Autodesk Inventor part; units mm, degrees
ref_plane "YZ Plane" through (0, 0, 0) normal (1, 0, 0) x (0, 1, 0)
ref_plane "XZ Plane" through (0, 0, 0) normal (0, 1, 0) x (-1, 0, 0)
ref_plane "XY Plane" through (0, 0, 0) normal (0, 0, 1) x (1, 0, 0)
sketch "Sketch3" plane through (0, 0, 0) normal (0, 0, 1) x (1, 0, 0)
  line L0 (-12.7, -19.05) -> (12.7, -19.05)
  line L1 (12.7, -19.05) -> (12.7, 19.05)
  line L2 (12.7, 19.05) -> (-12.7, 19.05)
  line L3 (-12.7, 19.05) -> (-12.7, -19.05)
  line L4 (-12.7, -19.05) -> (12.7, 19.05) construction
  line L5 (12.7, -19.05) -> (-12.7, 19.05) construction
  point P0 (0, 0)
  dimension "d0" = 25.4
  dimension "d1" = 38.1
extrude "Extrusion1" add sketch "Sketch3" along normal mid plane 12.7
sketch "Sketch4" plane through (0, 0, 6.35) normal (0, 0, 1) x (1, 0, 0)
  circle A0 centre (0, 0) radius 2.667
  dimension "d4" = 5.334
extrude "Extrusion2" cut sketch "Sketch4" against normal through all
sketch "Sketch5" plane through (-12.7, -19.05, 6.35) normal (-1, 0, 0) x (0, 0, 1)
  line L0 (3.175, 6.35) -> (50.8, 6.35)
  line L1 (-12.7, 38.1) -> (-12.7, 0)
  line L2 (0, 0) -> (0, 38.1)
  line L3 (-12.7, 0) -> (0, 0)
  line L4 (0, 0) -> (0, 6.35)
  line L5 (0, 6.35) -> (-12.7, 6.35)
  line L6 (-12.7, 6.35) -> (-12.7, 0)
  point P0 (-6.35, 19.05)
  point P1 (-12.7, 6.35)
  dimension "d9" = 6.35
extrude "Extrusion3" cut sketch "Sketch5" against normal through all
sketch "Sketch8" plane through (-12.7, -12.7, -6.35) normal (-1, 0, 0) x (0, 0, 1)
  line L0 (-4.7625, 21.8398) -> (-4.7625, 13.2284)
  line L1 (12.7, 0) -> (12.7, 31.75)
  line L2 (12.7, 0) -> (-4.7625, 0)
  line L3 (-4.7625, 0) -> (-4.7625, 31.75)
  line L4 (-4.7625, 31.75) -> (12.7, 31.75)
  line L5 (12.7, 31.75) -> (12.7, 0)
  point P0 (6.35, 12.7)
  point P1 (-4.7625, 13.2284)
extrude "Extrusion5" add sketch "Sketch8" along normal blind 6.35
mirror "Mirror1" about plane through (0, 0, 0) normal (1, 0, 0) of "Extrusion5"
sketch "Sketch6" plane through (0, 0, 0) normal (0, 0, 1) x (1, 0, 0)
  circle A0 centre (0, 25.4) radius 15.367
  point P0 (0, 0)
  dimension "d10" = 25.4
  dimension "d13" = 30.734
extrude "cutOutForGuide" cut sketch "Sketch6" along normal mid plane 11.0998
sketch "Sketch9" plane through (0, 0, 6.35) normal (0, 0, 1) x (1, 0, 0)
  circle A0 centre (0, 0) radius 3.1242
  dimension "d16" = 6.2484
extrude "Extrusion6" cut sketch "Sketch9" against normal blind 9.525
properties part number "preventWireJumpingSingleSupport" material "PBT Plastic"
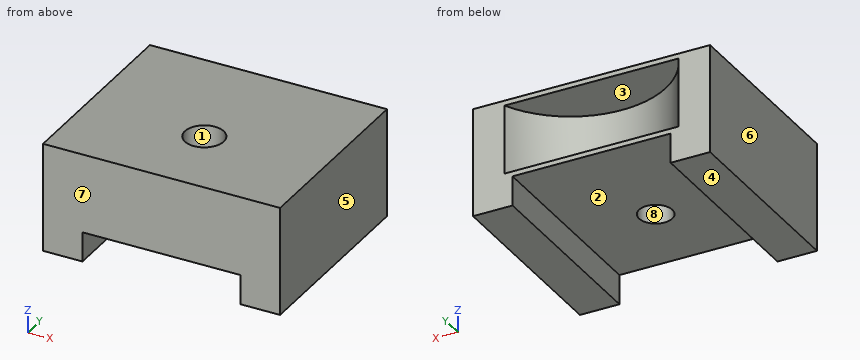
CAD build for the part. Positions are in the model's coordinates, mm. Face numbers are marked on the shaded views. A direction names the side the tool comes from. Round coordinates to 2 decimals unless told otherwise and drop trailing zeros. Write each loop counter-clockwise with the first axis right and the second up, starting at its lowest first coordinate (ties: lowest second). Pieces come first, ordered by that corner, then holes. Notation, with made-up numbers: (21.5, 8.25) - (40.5, 8.25) arc R15 cw to (40.5, 25.25) - close; hole circle Ø9 at (-27, 67). An arc over 180 degrees is marked (long way). Return JSON: item names as keys, results as strings. Group by question number.
Item 1: Mould opens along X. For the marked faces 5, 6, 7 and 8 say: +X half, -X half, draft (parallel to the pull), parting line (faces both ways), or undercut.
Item 2: Band-saw the part on D-D on z = -7.5. List the corners of the cut face in (x, y).
Item 3: Band-saw the part on C-C on z = -3.75. List the corners of the cut face in (x, y).
Item 4: Band-saw the part on A-A on x = 0. List the corners of the cut face in (y, z) (3 decimals).
Item 5: 3-axis set-ups, long thin cutter, end or side, ignore diameter. For the marked faces 1, 2, 3 and 4: which of +Z, -Z, +X, -X, +Y, -Y reach the whole face in a straight line?
Item 6: Probe probe 1 along Y at (x, z) = (0, 4.25); probe 2 along Z at (x, y) = (-3.5, -4); probe 3 along Y at (x, z) = (0, -4.75). List the from-to ranges inside material, lowest first.
Item 7: Flat gauge pins, fed straight in: pin 1 Ø3 at (x, z) = (-4.5, 0.5) entering from +Y; pin 2 Ø7 at (x, y) = (2, 16.5) entering from -Z; pin 3 Ø10 at (x, z) = (3, -0.5) entering from +Y. Where does each tip first touch, or does it go through?
Resolved:
{
 "1": {"face 5": "+X half", "face 6": "-X half", "face 7": "draft", "face 8": "undercut"},
 "2": {"outline": "(-19.05, -12.7) - (-12.7, -12.7) - (-12.7, 19.05) - (-19.05, 19.05) - close; (12.7, -12.7) - (19.05, -12.7) - (19.05, 19.05) - (12.7, 19.05) - close"},
 "3": {"outline": "(-19.05, -12.7) - (19.05, -12.7) - (19.05, 19.05) - (13.99, 19.05) arc R15.37 cw to (-13.99, 19.05) - (-19.05, 19.05) - close; hole circle Ø5.33 at (0, 0)"},
 "4": {"outline": "(-12.7, -6.35) - (-2.667, -6.35) - (-2.667, -3.175) - (-3.124, -3.175) - (-3.124, 6.35) - (-12.7, 6.35) - close; (2.667, -6.35) - (19.05, -6.35) - (19.05, -5.55) - (10.033, -5.55) - (10.033, 5.55) - (19.05, 5.55) - (19.05, 6.35) - (3.124, 6.35) - (3.124, -3.175) - (2.667, -3.175) - close"},
 "5": {"face 1": "+Z", "face 2": "-Z, +Y, -Y", "face 3": "+Y", "face 4": "-Z, +X, -X, +Y, -Y"},
 "6": {"probe 1": "y = -12.7 to -3.12, 3.12 to 10.03", "probe 2": "z = -6.35 to 6.35", "probe 3": "y = -12.7 to -2.67, 2.67 to 10.03"},
 "7": {"pin 1": "stops at y = 11.25", "pin 2": "stops at z = -6.35", "pin 3": "stops at y = 12.28"}
}
